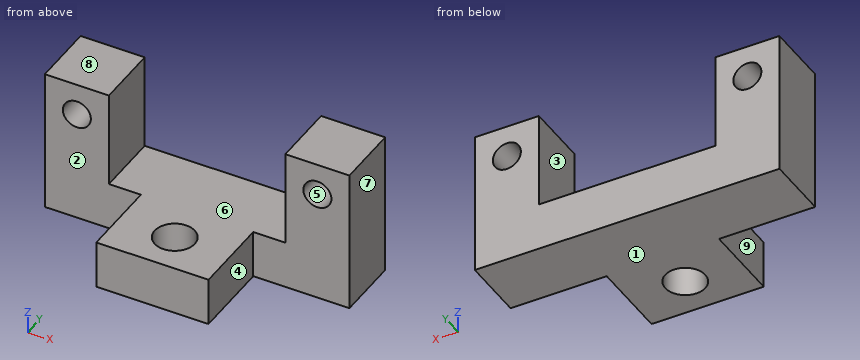
from build123d import *

# Parameters (mm, degrees)
F0_W     = 44.45
F0_H     = 31.75
F1_DEPTH = 19.05
F2_R     = 7.9375
F3_DEPTH = 19.051
F4_W     = 25.4
F4_H     = 25.4
F5_DEPTH = 38.1
F6_R     = 5.55625
F7_DEPTH = 25.401
F8_R     = 5.55625
F9_DEPTH = 25.401


with BuildPart() as f1:
    # F0 (on Top) → F1 (new body)
    with BuildSketch(Plane.XY):
        Polygon((68.285176, -9.157275), (-52.364824, -9.157275), (-52.364824, -34.557275), (-14.264824, -34.557275), (30.185176, -34.557275), (68.285176, -34.557275), align=None)
        with Locations((7.960176, -50.432275)):
            Rectangle(F0_W, F0_H)
    extrude(amount=F1_DEPTH)

    # F2 (on face) → F3 (cut, through all)
    with BuildSketch(Plane.XY.offset(19.05)):
        with Locations((7.960176, -50.432275)):
            Circle(F2_R)
    extrude(amount=-F3_DEPTH, mode=Mode.SUBTRACT)

    # F4 (on face) → F5 (join)
    with BuildSketch(Plane.XY.offset(19.05)):
        with Locations((-39.664824, -21.857275)):
            Rectangle(F4_W, F4_H)
        with Locations((55.585176, -21.857275)):
            Rectangle(F4_W, F4_H)
    extrude(amount=F5_DEPTH)

    # F6 (on face) → F7 (cut, through all)
    with BuildSketch(Plane.XZ.offset(34.557275)):
        with Locations((-39.664824, 44.45)):
            Circle(F6_R)
    extrude(amount=-F7_DEPTH, mode=Mode.SUBTRACT)

    # F8 (on face) → F9 (cut, through all)
    with BuildSketch(Plane.XZ.offset(34.557275)):
        with Locations((55.585176, 44.45)):
            Circle(F8_R)
    extrude(amount=-F9_DEPTH, mode=Mode.SUBTRACT)


solid = f1.part
Geometry: final body of the model. Coordinates: model frame, mm. Face numbers are marked on the shaded views. A direction names the side the tool comes from. Give positions to 0.01 mm unless a question says otherwise; leave off trailing zeros. Loops run counter-clockwise (first coordinate to the right, second up) from the corner with the lowest first, then second, coordinate; pieces in that order, holes last. Notation, with made-up numbers: (-20.5, 27) - (7.5, 27) arc R26 ccw to (7.5, 41) - close; hole circle Ø10 at (4.25, -28). An arc over 180 degrees is marked (long way). One line per question, with ' | ' between items. Start each with the question number.
(1) Reachability of the marked faces 1, 2, 3, 4 and 5 from +Z, -Z, +X, -X, +Y, -Y: full face, straight path, thin tool, end or side. Return the list, or none.
(2) Section query D-D on x = 4. Return loops of the section in (y, z).
(3) Section query A-A on z = 33. Return loops of the section in (x, y).
(4) Section query B-B on z = 44.45. Return loops of the section in (x, y), then the cut area to 3 significant figures.
(5) Contact query for flat-ended pins moving along their axis: pin 1 (10 mm diameter, centred on x = -8.5, y = -54, fed in from +Z); pin 2 (5.5 mm diameter, centred on y = -48.5, z = 5.5, fed in from +X); pin 3 (14.5 mm diameter, centred on x = 55.59, z = 44.45, fed in from -Y). Output: stop coordinate, or through.
(6) Section query C-C on y = -27.5. Return loops of the section in (x, z), then the cut area to 3 significant figures.
(7) Pull-direction query (X, two-part tool) for the marked faces 6, 7, 8 and 9; classes: released by +X, released by -X, zero draft, split by the parting line, or undercut.
(8) Ray query, line 1 (X direction, y = -24, z = 44); line 2 (X direction, y = -18, z = 31); line 3 (Z direction, x = -14, y = -29.5). Return the intervals inside material, ascending. Write a range as from..to.
The answers:
1) face 1: -Z, +X, -X, +Y, -Y | face 2: +Z, -Z, -X, -Y | face 3: +Z, +Y, -Y | face 4: +Z, -Z, +X, -Y | face 5: +Y, -Y
2) outline: (-66.31, 0) - (-57.31, 0) - (-57.31, 19.05) - (-66.31, 19.05) - close; (-43.55, 0) - (-9.16, 0) - (-9.16, 19.05) - (-43.55, 19.05) - close
3) outline: (-52.36, -34.56) - (-26.96, -34.56) - (-26.96, -9.16) - (-52.36, -9.16) - close; (42.89, -34.56) - (68.29, -34.56) - (68.29, -9.16) - (42.89, -9.16) - close
4) outline: (-52.36, -34.56) - (-45.22, -34.56) - (-45.22, -9.16) - (-52.36, -9.16) - close; (-34.11, -34.56) - (-26.96, -34.56) - (-26.96, -9.16) - (-34.11, -9.16) - close; (42.89, -34.56) - (50.03, -34.56) - (50.03, -9.16) - (42.89, -9.16) - close; (61.14, -34.56) - (68.29, -34.56) - (68.29, -9.16) - (61.14, -9.16) - close | area: 726 mm2
5) pin 1: z = 19.05 | pin 2: x = 30.19 | pin 3: y = -34.56
6) outline: (-52.36, 0) - (68.29, 0) - (68.29, 57.15) - (42.89, 57.15) - (42.89, 19.05) - (-26.96, 19.05) - (-26.96, 57.15) - (-52.36, 57.15) - close; hole circle Ø11.11 at (-39.66, 44.45); hole circle Ø11.11 at (55.59, 44.45) | area: 4,040 mm2
7) face 6: undercut | face 7: released by +X | face 8: zero draft | face 9: released by -X
8) line 1: -52.36..-45.2, -34.13..-26.96, 42.89..50.05, 61.12..68.29 | line 2: -52.36..-26.96, 42.89..68.29 | line 3: 0..19.05
